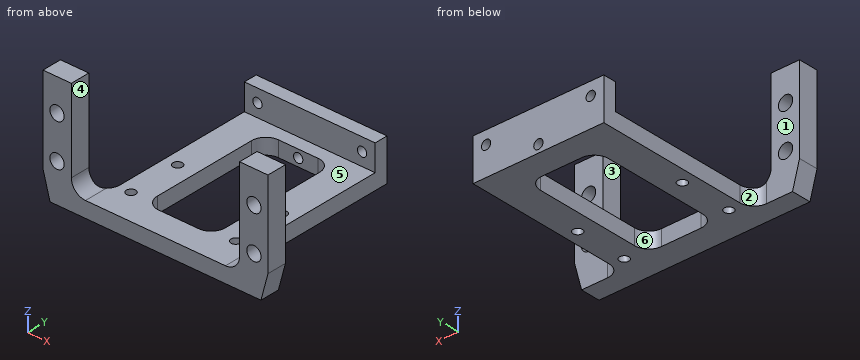
from build123d import *

# Parameters (mm, degrees)
F1_DEPTH  = 4.7625
F3_DEPTH  = 37.338
F4_R      = 3.429
F5_W      = 31.75
F5_H      = 6.35
F5_H_2    = 3.81
F6_DEPTH  = 3.2258
F8_D      = 3.4544
F10_D     = 2.2606
F10_DEPTH = 10.16
F10_TIP   = 0.6791527577
F12_DEPTH = 3.8110001
F14_D     = 2.2606


with BuildPart() as f1:
    # F0 (on Front) → F1 (new body)
    with BuildSketch(Plane.XZ):
        with BuildLine():
            Line((-25.6032, -13.6805935506), (0, -13.6805935506))
            Line((0, -13.6805935506), (25.6032, -13.6805935506))
            Line((25.6032, -13.6805935506), (27.305, -7.3305935506))
            Line((27.305, -7.3305935506), (27.305, 13.6805935506))
            Line((27.305, 13.6805935506), (20.4216, 13.6805935506))
            Line((20.4216, 13.6805935506), (20.4216, -6.4415935506))
            ThreePointArc((20.4216, -6.4415935506), (19.4172691527, -8.8662627033), (16.9926, -9.8705935506))
            Line((16.9926, -9.8705935506), (0, -9.8705935506))
            Line((0, -9.8705935506), (-16.9926, -9.8705935506))
            ThreePointArc((-16.9926, -9.8705935506), (-19.4172691527, -8.8662627033), (-20.4216, -6.4415935506))
            Line((-20.4216, -6.4415935506), (-20.4216, 13.6805935506))
            Line((-20.4216, 13.6805935506), (-27.305, 13.6805935506))
            Line((-27.305, 13.6805935506), (-27.305, -7.3305935506))
            Line((-27.305, -7.3305935506), (-25.6032, -13.6805935506))
        make_face()
    extrude(amount=F1_DEPTH)

    # F2 (on face) → F3 (join)
    with BuildSketch(Plane(origin=(0, 0, 0), x_dir=(-1, 0, 0), z_dir=(0, 1, 0))):
        Polygon((15.875, -9.8705935506), (0, -9.8705935506), (-15.875, -9.8705935506), (-15.875, -13.6805935506), (0, -13.6805935506), (15.875, -13.6805935506), align=None)
    extrude(amount=F3_DEPTH)

    # F4
    f4_edges = [f1.edges().sort_by_distance(p)[0] for p in [
        (15.875, 0, -11.775594),
        (-15.875, 0, -11.775594),
    ]]
    fillet(f4_edges, radius=F4_R)

    # F5 (on face) → F6 (join)
    with BuildSketch(Plane(origin=(0, 37.338, 0), x_dir=(-1, 0, 0), z_dir=(0, 1, 0))):
        with Locations((0, -6.6955935506)):
            Rectangle(F5_W, F5_H)
        with Locations((0, -11.7755935506)):
            Rectangle(F5_W, F5_H_2)
    extrude(amount=F6_DEPTH)

    # F8 (through all)
    with Locations(Plane(origin=(0, 0, 0), x_dir=(1, 0, 0), z_dir=(0, 1, 0))):
        with Locations((-23.9014, -5.8859053767), (-23.9014, 4.3248946233), (23.9014, 4.4349935506), (23.9014, -5.8859053767)):
            Hole(F8_D / 2)

    # F10
    with Locations(Plane(origin=(0, 40.5638, 0), x_dir=(-1, 0, 0), z_dir=(0, 1, 0))):
        with Locations((-12.7, -6.6955935506), (12.7, -6.6955935506), (0, -11.7755935506)):
            Hole(F10_D / 2, depth=F10_DEPTH)
            with Locations((0, 0, -(F10_DEPTH + F10_TIP / 2))):  # 118° drill point
                Cone(0, F10_D / 2, F10_TIP, mode=Mode.SUBTRACT)

    # F11 (on face) → F12 (cut, through all)
    with BuildSketch(Plane.XY.offset(-9.8705935506)):
        with BuildLine():
            Line((-4.826, 1.5875), (4.826, 1.5875))
            ThreePointArc((4.826, 1.5875), (7.2506691527, 2.5918308473), (8.255, 5.0165))
            Line((8.255, 5.0165), (8.255, 30.7467))
            ThreePointArc((8.255, 30.7467), (7.2506691527, 33.1713691527), (4.826, 34.1757))
            Line((4.826, 34.1757), (-4.826, 34.1757))
            ThreePointArc((-4.826, 34.1757), (-7.2506691527, 33.1713691527), (-8.255, 30.7467))
            Line((-8.255, 30.7467), (-8.255, 5.0165))
            ThreePointArc((-8.255, 5.0165), (-7.2506691527, 2.5918308473), (-4.826, 1.5875))
        make_face()
    extrude(amount=-F12_DEPTH, mode=Mode.SUBTRACT)

    # F14 (through all)
    with Locations(Plane.XY.offset(-9.8705935506)):
        with Locations((12.7, 2.8575), (12.7, 15.5575), (-12.7, 2.8575), (-12.7, 15.5575)):
            Hole(F14_D / 2)


solid = f1.part
Can you work these out from the model? Positions are in its coordinate system, mm. Face numbers are marked on the shaded views. A direction names the side the tool comes from. Give positions to 0.01 mm unless a question says otherwise; leave off trailing zeros. Loops run counter-clockwise (first coordinate to the right, second up) from the corner with the lowest first, then second, coordinate; pieces in that order, holes last. Notation, with made-up numbers: (27, 51) - (63, 51) arc R15 ccw to (63, 65) - close; hole circle Ø9 at (82.5, 48.25). An arc over 180 degrees is marked (long way). Answer as a JSON object with one key per item and string values.
Q1. Imagine slicing it at A-A on y = 23.5. Write out the boundary of the cut face in (x, z) (3 decimals).
Geometry says:
{"outline": "(-15.875, -13.681) - (-8.255, -13.681) - (-8.255, -9.871) - (-15.875, -9.871) - close; (8.255, -13.681) - (15.875, -13.681) - (15.875, -9.871) - (8.255, -9.871) - close"}
Q2. If we mould it in two halves opening along X, with no side actions, what happens to the marked faces 1, 2 and 3? For each: pulls with the +X half, pulls with the -X half, needs draft (parallel to the pull), parting line crosses it, or undercut.
Geometry says:
{"face 1": "needs draft", "face 2": "pulls with the -X half", "face 3": "undercut"}
Q3. If I drill on L1, parallel to Y at x = -12.7, z = -10.7; L2, parallel to Z at x = 23.5, y = -3; L3, parallel to X at y = 15, z = -10.5 (3 decimals), over which ranges is the centre line in solid material (lowest first)?
Geometry says:
{"L1": "-4.76 to 1.73, 3.99 to 14.43, 16.69 to 40.56", "L2": "-13.68 to -6.11, -2.76 to 4.21, 7.57 to 13.68", "L3": "-15.875 to -13.683, -11.717 to -8.255, 8.255 to 11.717, 13.683 to 15.875"}
Q4. Imagine slicing it at D-D on x = 12.7. Write out the boundary of the cut face in (y, z).
Geometry says:
{"outline": "(-4.76, -13.68) - (1.73, -13.68) - (1.73, -9.87) - (-4.76, -9.87) - close; (3.99, -13.68) - (14.43, -13.68) - (14.43, -9.87) - (3.99, -9.87) - close; (16.69, -13.68) - (40.56, -13.68) - (40.56, -7.83) - (37.34, -7.83) - (37.34, -9.87) - (16.69, -9.87) - close; (37.34, -5.57) - (40.56, -5.57) - (40.56, -3.52) - (37.34, -3.52) - close"}
Q5. Imagine slicing it at B-B on x = 3. Write out the boundary of the cut face in (y, z), plus the area to 3 significant figures.
Geometry says:
{"outline": "(-4.76, -13.68) - (1.59, -13.68) - (1.59, -9.87) - (-4.76, -9.87) - close; (34.18, -13.68) - (40.56, -13.68) - (40.56, -3.52) - (37.34, -3.52) - (37.34, -9.87) - (34.18, -9.87) - close", "area": "69.0 mm²"}
Q6. Imagine slicing it at C-C on z = -1.25. Write out the boundary of the cut face in (x, y) (1 decimal).
Geometry says:
{"outline": "(-27.3, -4.8) - (-20.4, -4.8) - (-20.4, 0) - (-27.3, 0) - close; (20.4, -4.8) - (27.3, -4.8) - (27.3, 0) - (20.4, 0) - close"}
Q7. Which directions (+Z, -Z, +X, -X, +Y, -Y) give clear straight access to the entire face, cutting with the end or side of a thin tool? Please do the marked faces 4, 5 and 6.
Geometry says:
{"face 4": "+Z, +Y, -Y", "face 5": "+Z, -Y", "face 6": "+Z, -Z"}
Q8. Will these pins go through, and if not, where does the flat tip stop? P1, Ø1, axis at x = -8.5, y = 8.5, coming from the +Z side; P2, Ø5, axis at y = 22.5, z = -9.5, coming from the -X side (3 decimals); P3, Ø3, axis at x = 23.9, z = -4.43, coming from the -Y side; P4, Ø10, axis at y = 29, z = -6, coming from the +X side (3 decimals).
Geometry says:
{"P1": "z = -9.87", "P2": "x = -15.875", "P3": "through", "P4": "x = 15.875"}
